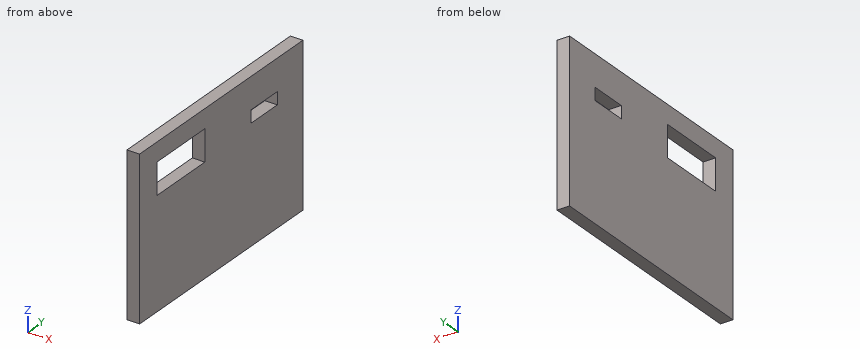
from build123d import *

# Parameters (mm, degrees)
F0_W     = 37.56
F0_H     = 25.4
F0_W_2   = 11
F0_H_2   = 5
F0_W_3   = 6
F0_H_3   = 2
F1_DEPTH = 2


with BuildPart() as f1:
    # F0 (on Right) → F1 (new body)
    with BuildSketch(Plane.YZ):
        with Locations((18.78, 12.7)):
            Rectangle(F0_W, F0_H)
        with Locations((9.5, 19.9)):
            Rectangle(F0_W_2, F0_H_2, mode=Mode.SUBTRACT)
        with Locations((28.67, 19.4)):
            Rectangle(F0_W_3, F0_H_3, mode=Mode.SUBTRACT)
    extrude(amount=F1_DEPTH)


solid = f1.part
Read the model definition and answer for the solid it produces. Units are mm, in the model's axes. Round coordinates to 2 decimals unless told otherwise and drop trailing zeros. Write each loop counter-clockwise with the first axis right and the second up, starting at its lowest first coordinate (ties: lowest second). Pieces come first, ordered by that corner, then holes.
1. Given pin 1 Ø10 at (y, z) = (21.5, 13) entering from -X, flat-ended and moving along its own axis, determine where the tip first touches the part or whether it passes through.
2. Straight lines are drawn through the part: L1, parallel to Y at x = 1.25, z = 18.5; L2, parallel to Y at x = 1.8, z = 22; L3, parallel to Z at x = 1.7, y = 13. For each, find the intervals that lie inside material, in ascending order.
3. The part is cut by section A-A, the plane z = 21.5. Determine the outline of the cut face in (x, y).
4. The part is cut by section B-B, the plane y = 29. Determine the outline of the cut face in (x, z).
5. The part is cut by section C-C, the plane x = 0.6. Determine the outline of the cut face in (y, z), then the cut area to 3 significant figures.
Values:
1. pin 1: stops at x = 0
2. L1: y = 0 to 4, 15 to 25.67, 31.67 to 37.56
2. L2: y = 0 to 4, 15 to 37.56
2. L3: z = 0 to 17.4, 22.4 to 25.4
3. outline: (0, 0) - (2, 0) - (2, 4) - (0, 4) - close; (0, 15) - (2, 15) - (2, 37.56) - (0, 37.56) - close
4. outline: (0, 0) - (2, 0) - (2, 18.4) - (0, 18.4) - close; (0, 20.4) - (2, 20.4) - (2, 25.4) - (0, 25.4) - close
5. outline: (0, 0) - (37.56, 0) - (37.56, 25.4) - (0, 25.4) - close; hole (4, 17.4) - (15, 17.4) - (15, 22.4) - (4, 22.4) - close; hole (25.67, 18.4) - (31.67, 18.4) - (31.67, 20.4) - (25.67, 20.4) - close
5. area: 887 mm2
